Could you check a few things on this model? Use its own coordinates, in mm. A direction names the side the tool comes from. Give positions to 0.01 mm unless a question says otherwise; leave off trailing zeros. Order: outer loops, then holes, each group sorted by start corner. A loop starts at its lowest first (then second) coordinate and runs counter-clockwise, first axis right, second up.
from build123d import *

# Parameters (mm, degrees)
ESQUISSE1_R               = 3.5
ESQUISSE1_W               = 3
ESQUISSE1_H               = 5.702159315
T_LE_DE_BASE_PLI_E1_DEPTH = 3


# Sheet-metal steps are written as plain solids
with BuildPart() as part:
    # Esquisse1 → Tôle de base pliée1 (new body)
    with BuildSketch(Plane.XY):
        Polygon((29.5, 47.5), (29.5, 37.5), (26.5, 37.5), (26.5, 47.5), (3, 47.5), (3, 46), (0, 46), (0, 41), (3, 41), (3, 38), (0, 38), (0, 33), (3, 33), (3, 14), (0, 14), (0, 1.5), (3, 1.5), (3, 0), (19.6, 0), (19.6, -3.5), (22.6, -3.5), (22.6, 0), (26.5, 0), (26.5, 2.7), (29.5, 2.7), (29.5, 0), (48.5, 0), (48.5, 1.5), (51.5, 1.5), (51.5, 11.2), (48.5, 11.2), (48.5, 31.2), (51.5, 31.2), (51.5, 46), (48.5, 46), (48.5, 47.5), align=None)
        with Locations((25.6, 24)):
            Circle(ESQUISSE1_R, mode=Mode.SUBTRACT)
        with BuildLine():
            Line((35.55, 25), (40.05, 25))
            ThreePointArc((40.05, 25), (41.05, 24), (40.05, 23))
            Line((40.05, 23), (35.55, 23))
            ThreePointArc((35.55, 23), (34.55, 24), (35.55, 25))
        make_face(mode=Mode.SUBTRACT)
        with BuildLine():
            Line((11.15, 25), (15.65, 25))
            ThreePointArc((15.65, 25), (16.65, 24), (15.65, 23))
            Line((15.65, 23), (11.15, 23))
            ThreePointArc((11.15, 23), (10.15, 24), (11.15, 25))
        make_face(mode=Mode.SUBTRACT)
        with Locations((28, 6.548920343)):
            Rectangle(ESQUISSE1_W, ESQUISSE1_H, mode=Mode.SUBTRACT)
    extrude(amount=-T_LE_DE_BASE_PLI_E1_DEPTH)


solid = part.part
Item 1: For faces 4 (the flat face through (26.5, 7, -1)), 5 (the flat face through (39, 0, -1)), 6 (the flat face through (26.5, 1, -1)), which set-ups out of +Z, -Z, +X, -X, +Y, -Y let a thin tool reach every point of the face, with its end or its side?
Findings:
face 4: +Z, -Z
face 5: +Z, -Z, +X, -Y
face 6: +Z, -Z, -Y
Item 2: Imagine slicing it at C-C on y = 24. List the corners of the cut face in (x, z) for me, then the cut area to 3 significant figures.
Findings:
outline: (3, -3) - (10.15, -3) - (10.15, 0) - (3, 0) - close; (16.65, -3) - (22.1, -3) - (22.1, 0) - (16.65, 0) - close; (29.1, -3) - (34.55, -3) - (34.55, 0) - (29.1, 0) - close; (41.05, -3) - (48.5, -3) - (48.5, 0) - (41.05, 0) - close
area: 76.5 mm2
Item 3: Imagine slicing it at D-D on z = -2.5. Give the number of separate pieces and of enclosed holes in the cut face, then the cut area to 3 significant figures.
Findings:
separate pieces: 1
enclosed holes: 4
area: 2,190 mm2
Item 4: Please list where these lines run through material, in increasing order: line 1 along Y through (x, z) = (25.6, -1.75); line 2 along Y through (x, z) = (35.5, -2.35); line 3 along X through (y, z) = (41.5, -2.5).
Findings:
line 1: y = 0 to 20.5, 27.5 to 47.5
line 2: y = 0 to 23, 25 to 47.5
line 3: x = 0 to 26.5, 29.5 to 51.5
Item 5: Imagine slicing it at A-A on y = 39. List the corners of the cut face in (x, z) for me.
Findings:
outline: (3, -3) - (26.5, -3) - (26.5, 0) - (3, 0) - close; (29.5, -3) - (51.5, -3) - (51.5, 0) - (29.5, 0) - close
Item 6: We'd pull the mould along Y, two halves only. Please class faces 1 (the flat face through (22.6, -2, -1)), 2 (the flat face through (28, 9.4, -1)), 3 (the flat face through (50, 1.5, -1)): +Y half, -Y half, draft (parallel to the pull), parting line (faces both ways), or undercut.
Findings:
face 1: draft
face 2: undercut
face 3: -Y half
Item 7: Imagine slicing it at B-B on x = 25.6. List the corners of the cut face in (y, z) for me.
Findings:
outline: (0, -3) - (20.5, -3) - (20.5, 0) - (0, 0) - close; (27.5, -3) - (47.5, -3) - (47.5, 0) - (27.5, 0) - close
Item 8: For pin 1 (9 mm diameter, centred on x = 25.6, y = 24, fed in from +Z); pin 2 (1.5 mm diameter, centred on x = 1, z = -2, fed in from -Y); pin 3 (1.5 mm diameter, centred on y = 26, z = -1, fed in from +X); pin 4 (0.9 mm diameter, centred on x = 28.5, z = -2, fed in from -Y), each with a flat end and sliding along its axis, tell me the tip position at first contact or that it passes through.
Findings:
pin 1: stops at z = 0
pin 2: stops at y = 1.5
pin 3: stops at x = 48.5
pin 4: stops at y = 2.7
